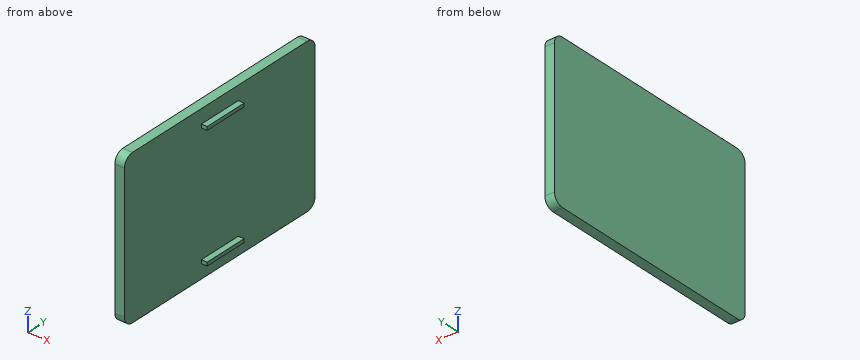
from build123d import *

# Parameters (mm, degrees)
SKETCH1_W           = 80
SKETCH1_H           = 120
BOSS_EXTRUDE1_DEPTH = 5
FILLET1_R           = 5
SKETCH2_W           = 1.804418344
SKETCH2_H           = 23.230636126
BOSS_EXTRUDE2_DEPTH = 3


with BuildPart() as part:
    # Sketch1 → Boss-Extrude1 (new body)
    with BuildSketch(Plane(origin=(0, 0, 0), x_dir=(0, 0, -1), z_dir=(1, 0, 0))):
        Rectangle(SKETCH1_W, SKETCH1_H)
    extrude(amount=BOSS_EXTRUDE1_DEPTH)

    # Fillet1
    fillet1_edges = [part.edges().sort_by_distance(p)[0] for p in [
        (2.5, -60, -40),
        (2.5, -60, 40),
        (2.5, 60, 40),
        (2.5, 60, -40),
    ]]
    fillet(fillet1_edges, radius=FILLET1_R)

    # Sketch2 → Boss-Extrude2 (add)
    with BuildSketch(Plane(origin=(5, 0, 0), x_dir=(0, 0, -1), z_dir=(1, 0, 0))):
        with Locations((-31.82671961, 0)):
            Rectangle(SKETCH2_W, SKETCH2_H)
    boss_extrude2 = extrude(amount=BOSS_EXTRUDE2_DEPTH)

    # Mirror1: Boss-Extrude2 across plane
    add(boss_extrude2.mirror(Plane.XY))


solid = part.part
Verification items for the finished model (mm, model axes). Coordinates: 2 decimals unless noted, no trailing zeros. Order: outer loops, then holes, each group sorted by start corner. A loop starts at its lowest first (then second) coordinate and runs counter-clockwise, first axis right, second up.
1. Scan lines: line 1 (X direction, y = 40, z = 35.5); line 2 (Y direction, x = 6.25, z = 32.5); line 3 (Y direction, x = 1.25, z = 36). Record each from-to range of solid material in increasing order.
Results found:
line 1: x = 0 to 5
line 2: y = -11.62 to 11.62
line 3: y = -59.9 to 59.9
2. Sectioned sample at A-A, the plane y = -9.5. Record the cut outline in (x, z).
Results found:
outline: (0, -40) - (5, -40) - (5, -32.73) - (8, -32.73) - (8, -30.92) - (5, -30.92) - (5, 30.92) - (8, 30.92) - (8, 32.73) - (5, 32.73) - (5, 40) - (0, 40) - close
3. Go/stop test with flat-tipped pins: pin 1 Ø12 at (y, z) = (26.5, 0) entering from +X; pin 2 Ø2.5 at (x, y) = (6.5, 5.5) entering from +Z; pin 3 Ø1.5 at (x, y) = (6.5, 5.5) entering from -Z. Record where each tip stops, or that it passes through.
Results found:
pin 1: stops at x = 5
pin 2: stops at z = 32.73
pin 3: stops at z = -32.73
4. Sectioned sample at B-B, the plane z = -19. Record the cut outline in (x, y), and give its area (3 significant figures).
Results found:
outline: (0, -60) - (5, -60) - (5, 60) - (0, 60) - close
area: 600 mm2
